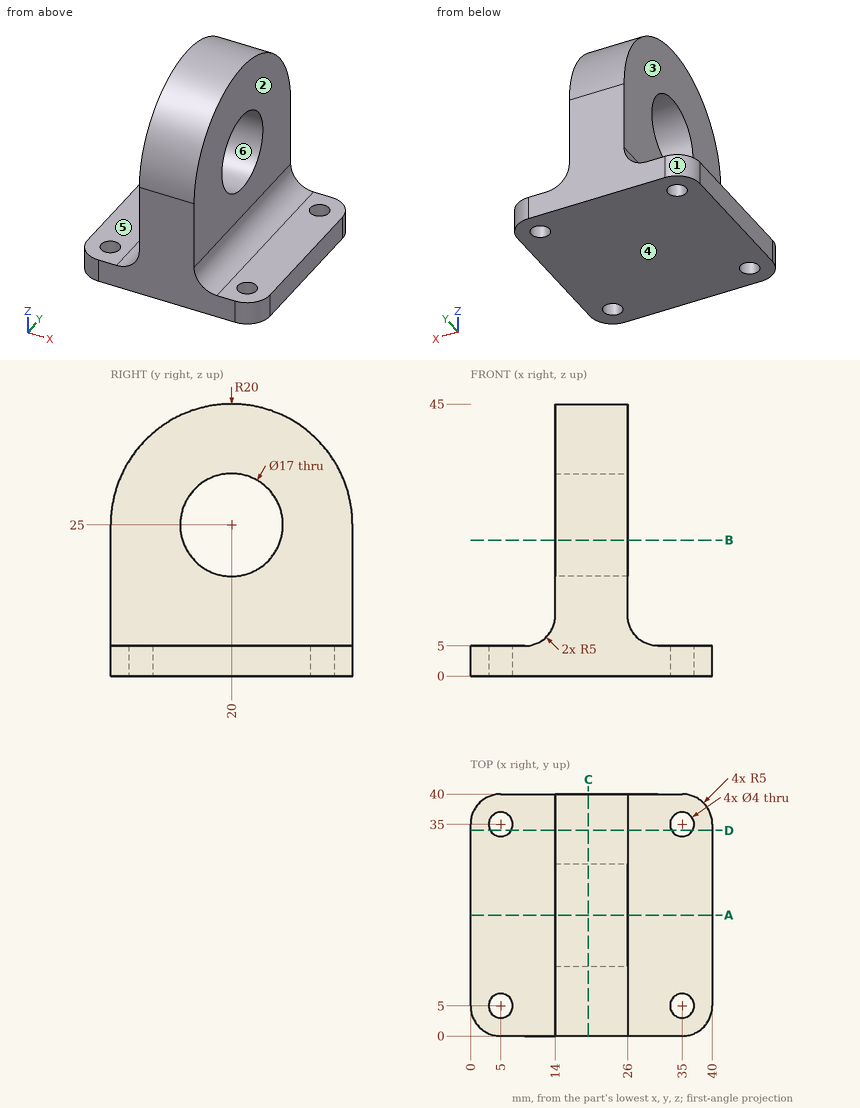
Input: dimensioned drawing with shaded views. Units: mm. Origin: part minimum x, y, z. A direction names the side the tool comes from. Coordinates: 2 decimals unless noted, no trailing zeros. Write each loop counter-clockwise with the first axis right and the second up, starting at its lowest first coordinate (ties: lowest second). Pieces come first, ordered by that corner, then holes. Notation, with made-up numbers: M -37.75,-18 L -6.75,-18 A21 ccw -6.75,18 Z; hole C 86.5,65.5 d3. An arc over 180 degrees is marked long. Use a Markdown table: item, result.
1) Section B-B, the plane z = 22.5. Output: boundary loops of the cut face in (x, y).
Conclusion:
| item | result |
|---|---|
| outline | M 14,0 L 26,0 L 26,11.88 L 14,11.88 Z; M 14,28.12 L 26,28.12 L 26,40 L 14,40 Z |
2) Mould query, pull axis Z, two halves, no side actions, for the marked faces 4, 5 and 6. Classes: pulls with the +Z half, pulls with the -Z half, needs draft (parallel to the pull), parting line crosses it, or undercut.
Conclusion:
| item | result |
|---|---|
| face 4 | pulls with the -Z half |
| face 5 | pulls with the +Z half |
| face 6 | undercut |
3) Section A-A, the plane y = 20. Output: boundary loops of the cut face in (x, z).
Conclusion:
| item | result |
|---|---|
| outline | M 0,0 L 40,0 L 40,5 L 31,5 A5 cw 26,10 L 26,16.5 L 14,16.5 L 14,10 A5 cw 9,5 L 0,5 Z; M 14,33.5 L 26,33.5 L 26,45 L 14,45 Z |
4) Ray query, L1, parallel to Y at x = 5, z = 2.05; L2, parallel to Z at x = 21.5, y = 20.5; L3, parallel to Y at x = 22, z = 25. Return the intervals inside material, ascending.
Conclusion:
| item | result |
|---|---|
| L1 | y = 0 to 3, 7 to 33, 37 to 40 |
| L2 | z = 0 to 16.51, 33.49 to 44.99 |
| L3 | y = 0 to 11.5, 28.5 to 40 |
5) Reachability of the marked faces 1, 2 and 3 from +Z, -Z, +X, -X, +Y, -Y: full face, straight path, thin tool, end or side. Return the list, or none.
Conclusion:
| item | result |
|---|---|
| face 1 | +Z, -Z, -X, +Y |
| face 2 | +Z, +X, +Y, -Y |
| face 3 | +Z, -X, +Y, -Y |
6) Section D-D, the plane y = 34. Output: boundary loops of the cut face in (x, z), then the cut area to 3 significant figures.
Conclusion:
| item | result |
|---|---|
| outline | M 0,0 L 3.27,0 L 3.27,5 L 0,5 Z; M 6.73,0 L 33.27,0 L 33.27,5 L 31,5 A5 cw 26,10 L 26,39.28 L 14,39.28 L 14,10 A5 cw 9,5 L 6.73,5 Z; M 36.73,0 L 40,0 L 40,5 L 36.73,5 Z |
| area | 587 mm^2 |
7) Section C-C, the plane x = 19.5. Output: boundary loops of the cut face in (y, z).
Conclusion:
| item | result |
|---|---|
| outline | M 0,0 L 40,0 L 40,25 A20 ccw 0,25 Z; hole C 20,25 d17 |
8) First-contact query: pin 1 Ø3 at (x, y) = (5, 35) entering from +Z; pin 2 Ø1 at (x, y) = (20.5, 16) entering from -Z; pin 3 Ø3 at (y, z) = (7, 11) entering from +X; pin 4 Ø17.5 at (y, z) = (23.5, 30.5) entering from -X. Flat tips, straight axial feed; report the tip coordinate or a pass-through.
Conclusion:
| item | result |
|---|---|
| pin 1 | passes through |
| pin 2 | stops at z = 0 |
| pin 3 | stops at x = 26.03 |
| pin 4 | stops at x = 14 |
